Geometry: final body of the model. Coordinates: model frame, mm. A direction names the side the tool comes from. Give positions to 0.01 mm unless a question says otherwise; leave off trailing zeros. Order: outer loops, then holes, each group sorted by start corner. A loop starts at its lowest first (then second) coordinate and runs counter-clockwise, first axis right, second up. Notation, with made-up numbers: (1.5, 31.5) - (38.5, 31.5) arc R12 cw to (38.5, 42.5) - close; hole circle Ø3 at (2, 53.5). An arc over 180 degrees is marked (long way). Put each result on its own line as item: value. Start each with the question number.
1. Section A-A on y = 4.5. Return the cut outline in (x, z), plus the area to 3 significant figures.
2. Ray query, line 1 along Y through (x, z) = (-16.5, 281.5) (3 decimals); line 2 along Z through (x, y) = (0, 5.5); line 3 along Z through (x, y) = (7.5, 3). Return the intervals inside material, ascending. Write a range as from..to.
3. Set-up query: faces 1 (the flat face through (-5, 9.652, 282)), 2 (the flat face through (72.12, -0.05, 269.16)). Return all of +Z, -Z, +X, -X, +Y, -Y with unobstructed straight access to the full face (end or side cutting, diameter ignored); none if empty.
4. First-contact query: P1, Ø1.5, axis at x = -5, y = -2.5, coming from the -Z side; P2, Ø4, axis at x = 13, z = 276, coming from the +Y side; P3, Ø3.5, axis at x = 11, z = 278.5, coming from the -Y side. Flat tips, straight axial feed; report the tip coordinate or a pass-through.
5. Mould query, pull axis Y, two halves, no side actions, for faces 3 (the flat face through (-72.12, -0.05, 269.16)), 4 (the flat face through (0, 10.795, 281)), 5 (the cylindrical face through (-1.022, -0.108, 278.916)). Classes: pulls with the +Y half, pulls with the -Y half, needs draft (parallel to the pull), parting line crosses it, or undercut.
from build123d import *

# Parameters (mm, degrees)
F3_ANGLE = 30


with BuildPart() as f3:
    # F1 (on Right) → F3 (revolve, symmetric)
    with BuildSketch(Plane.YZ) as f3_sk:
        with BuildLine():
            ThreePointArc((-10.795, 280.8224), (-9.902261, 278.667139), (-7.747, 277.7744))
            Line((-7.747, 277.7744), (7.747, 277.7744))
            ThreePointArc((7.747, 277.7744), (9.902261, 278.667139), (10.795, 280.8224))
            Line((10.795, 280.8224), (10.795, 282.9814))
            Line((10.795, 282.9814), (9.652, 282.9814))
            Line((9.652, 282.9814), (9.652, 280.8224))
            ThreePointArc((9.652, 280.8224), (9.094038, 279.475362), (7.747, 278.9174))
            Line((7.747, 278.9174), (-7.747, 278.9174))
            ThreePointArc((-7.747, 278.9174), (-9.094038, 279.475362), (-9.652, 280.8224))
            Line((-9.652, 280.8224), (-9.652, 282.9814))
            Line((-9.652, 282.9814), (-10.795, 282.9814))
            Line((-10.795, 282.9814), (-10.795, 280.8224))
        make_face()
    revolve(axis=Axis((0, -102.103345, 0), (0, -1, 0)), revolution_arc=F3_ANGLE / 2)
    revolve(f3_sk.sketch, axis=Axis((0, -102.103345, 0), (0, 1, 0)), revolution_arc=F3_ANGLE / 2)


solid = f3.part
Resolved:
1. outline: (-72.19, 269.41) - (-71.89, 268.31) arc R277.77 cw to (71.89, 268.31) - (72.19, 269.41) arc R278.92 ccw to start
1. area: 167 mm^2
2. line 1: -10.795..-9.652, 9.652..10.795
2. line 2: 277.77..278.92
2. line 3: 277.67..278.82
3. face 1: +Z
3. face 2: -Z, +X, +Y, -Y
4. P1: z = 277.71
4. P2: y = 9.47
4. P3: y = -10.77
5. face 3: needs draft
5. face 4: pulls with the +Y half
5. face 5: undercut
